CAD build for the part. Positions are in the model's coordinates, mm. A direction names the side the tool comes from. Coordinates: 2 decimals unless noted, no trailing zeros. Write each loop counter-clockwise with the first axis right and the second up, starting at its lowest first coordinate (ties: lowest second). Pieces come first, ordered by that corner, then holes. Notation, with made-up numbers: M 50.5,50.25 L 108.5,50.25 A16 ccw 108.5,74.25 Z; hole C 49.25,14.5 d3. An arc over 180 degrees is marked long. Put each result on its own line as item: value. Start each with the question number.
```python
from build123d import *

# Parameters (mm, degrees)
SKETCH1_W      = 647.7
SKETCH1_H      = 508
SKETCH1_W_2    = 596.9
SKETCH1_H_2    = 457.2
EXTRUDE1_DEPTH = 13.208
FILLET1_R      = 6.35


with BuildPart() as part:
    # Sketch1 → Extrude1 (new body)
    with BuildSketch(Plane.XY):
        Rectangle(SKETCH1_W, SKETCH1_H)
        Rectangle(SKETCH1_W_2, SKETCH1_H_2, mode=Mode.SUBTRACT)
    extrude(amount=-EXTRUDE1_DEPTH)

    # Fillet1
    fillet1_edges = [part.edges().sort_by_distance(p)[0] for p in [
        (323.85, 254, -6.604),
        (323.85, -254, -6.604),
        (-323.85, -254, -6.604),
        (-323.85, 254, -6.604),
    ]]
    fillet(fillet1_edges, radius=FILLET1_R)


solid = part.part
```
(1) Slice it at A-A, the plane y = -64. Write the cut outline in (x, z).
(2) Two-plate mould, pull along X, no slides. Class faces 3 (the face through (-298.45, -3, -7)), 4 (the face through (323.85, -3, -7)), 5 (the face through (-323.85, -3, -7)), 6 (the face through (-4, 254, -7)): +X half, -X half, draft (parallel to the pull), parting line (faces both ways), or undercut.
(3) Slice it at B-B, the plane z = -5. Write the cut outline in (x, y).
(4) Which spindle directions (+Z, -Z, +X, -X, +Y, -Y) get a long thin tool onto all of the face, cutting with end or side? Do faces 1 (the face through (-4, -254, -7)), 2 (the face through (-4, 228.6, -7)). Say none if no direction does.
(5) Drill centre lines: line 1 (X direction, y = 113, z = -3); line 2 (Y direction, x = -26, z = -7). Where is each one in solid material? Low to high. Write a range as [from, to].
(6) Slice it at C-C, the plane x = -246. Write the cut outline in (y, z).
Result set:
1. outline: M -323.85,-13.21 L -298.45,-13.21 L -298.45,0 L -323.85,0 Z; M 298.45,-13.21 L 323.85,-13.21 L 323.85,0 L 298.45,0 Z
2. face 3: undercut
2. face 4: +X half
2. face 5: -X half
2. face 6: draft
3. outline: M -323.85,-247.65 A6.35 ccw -317.5,-254 L 317.5,-254 A6.35 ccw 323.85,-247.65 L 323.85,247.65 A6.35 ccw 317.5,254 L -317.5,254 A6.35 ccw -323.85,247.65 Z; hole M -298.45,-228.6 L 298.45,-228.6 L 298.45,228.6 L -298.45,228.6 Z
4. face 1: +Z, -Z, +X, -X, -Y
4. face 2: +Z, -Z
5. line 1: x = [-323.85, -298.45], [298.45, 323.85]
5. line 2: y = [-254, -228.6], [228.6, 254]
6. outline: M -254,-13.21 L -228.6,-13.21 L -228.6,0 L -254,0 Z; M 228.6,-13.21 L 254,-13.21 L 254,0 L 228.6,0 Z
